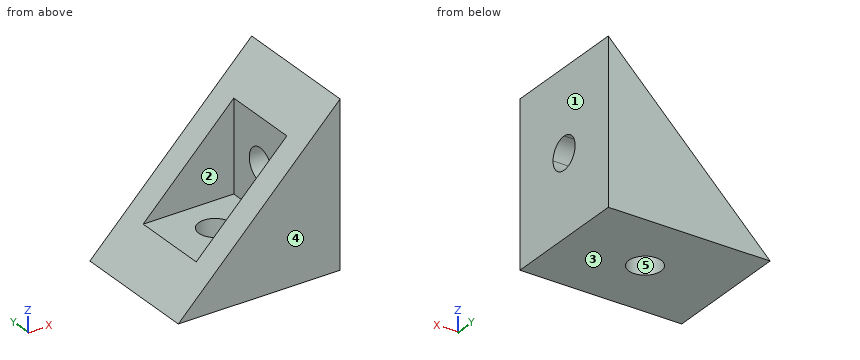
```python
from build123d import *

# Parameters (mm, degrees)
F1_DEPTH = 20
F2_DEPTH = 4
F4_DEPTH = 4
F6_DEPTH = 25.4
F7_R     = 2.5
F8_DEPTH = 25.4


with BuildPart() as f1:
    # F0 (on Front) → F1 (new body)
    with BuildSketch(Plane.XZ):
        Polygon((-7, -7), (-12.5, -12.5), (7, -12.5), (12.5, -12.5), (12.5, -7), (12.5, 12.5), (7, 7), (7, -7), align=None)
    extrude(amount=F1_DEPTH)

    # F0 (on Front) → F2 (join)
    with BuildSketch(Plane.XZ):
        Polygon((-7, -7), (-12.5, -12.5), (7, -12.5), (12.5, -12.5), (12.5, -7), (12.5, 12.5), (7, 7), (7, -7), align=None)
        Polygon((7, 7), (-7, -7), (7, -7), align=None)
    extrude(amount=F2_DEPTH)

    # F3 (on face) → F4 (join)
    with BuildSketch(Plane.XZ.offset(20)):
        Polygon((12.5, 12.5), (-12.5, -12.5), (12.5, -12.5), align=None)
    extrude(amount=-F4_DEPTH)

    # F5 (on face) → F6 (cut)
    with BuildSketch(Plane(origin=(7, 0, 0), x_dir=(0, -1, 0), z_dir=(-1, 0, 0))):
        with BuildLine():
            Line((10, 2.5), (10, -2.5))
            ThreePointArc((10, -2.5), (11.767767, -1.767767), (12.5, 0))
            ThreePointArc((12.5, 0), (11.767767, 1.767767), (10, 2.5))
        make_face()
        with BuildLine():
            ThreePointArc((10, 2.5), (7.5, 0), (10, -2.5))
            Line((10, -2.5), (10, 2.5))
        make_face()
    extrude(amount=-F6_DEPTH, mode=Mode.SUBTRACT)

    # F7 (on face) → F8 (cut)
    with BuildSketch(Plane.XY.offset(-7)):
        with Locations((0, -10)):
            Circle(F7_R)
    extrude(amount=-F8_DEPTH, mode=Mode.SUBTRACT)


solid = f1.part
```
The model under review builds one solid part; all positions refer to its coordinate system, in mm. Face numbers are marked on the shaded views. A direction names the side the tool comes from. Round coordinates to 2 decimals unless told otherwise and drop trailing zeros. Loops run counter-clockwise (first coordinate to the right, second up) from the corner with the lowest first, then second, coordinate; pieces in that order, holes last. Notation, with made-up numbers: M 70,-38.75 L 120,-38.75 A25 ccw 120,-24.75 Z; hole C 19.5,-11 d1. An arc over 180 degrees is marked long. Write item = value, one per line.
Item 1: Machinability: for the marked faces 1 and 2, which of the approach directions +Z, -Z, +X, -X, +Y, -Y give a long, thin tool a straight path to every point of the face, cutting with its end or side? Answer none if there is none.
Return value:
face_1 = +Z, -Z, +X, +Y, -Y
face_2 = +Z, -X
Item 2: Take a section at B-B on y = -9.5. Write out the cut boundary in (x, z), then the cut area to 3 significant figures.
Return value:
outline = M -12.5,-12.5 L -2.45,-12.5 L -2.45,-7 L -7,-7 Z; M 2.45,-12.5 L 12.5,-12.5 L 12.5,-2.45 L 7,-2.45 L 7,-7 L 2.45,-7 Z; M 7,2.45 L 12.5,2.45 L 12.5,12.5 L 7,7 Z
area = 161 mm2
Item 3: For line 1 (Y direction, x = 2.5, z = -2); line 2 (Y direction, x = 0, z = -11.15); line 3 (X direction, y = -7.25, z = -2), list the stretches that pass through material, from the lowest coordinate up. Write a range as [from, to].
Return value:
line_1 = [-20, -16], [-4, 0]
line_2 = [-20, -12.5], [-7.5, 0]
line_3 = [7, 12.5]
Item 4: Take a section at D-D on x = 5. Write out the cut boundary in (y, z), then the cut area to 3 significant figures.
Return value:
outline = M -20,-12.5 L 0,-12.5 L 0,5 L -4,5 L -4,-7 L -16,-7 L -16,5 L -20,5 Z
area = 206 mm2
Item 5: The part is to be moulded in two halves that separate along Y. For the marked faces 3, 4 and 5, say which applies: released by +Y, released by -Y, zero draft, split by the parting line, or undercut.
Return value:
face_3 = zero draft
face_4 = released by -Y
face_5 = undercut
Item 6: Take a section at A-A on x = 0. Write out the cut boundary in (y, z), then the cut area to 4 significant figures.
Return value:
outline = M -20,-12.5 L -12.5,-12.5 L -12.5,-7 L -16,-7 L -16,0 L -20,0 Z; M -7.5,-12.5 L 0,-12.5 L 0,0 L -4,0 L -4,-7 L -7.5,-7 Z
area = 138.5 mm2
Item 7: Insertion check: P1, Ø12, axis at x = -3, z = 3.5, coming from the -Y side; P2, Ø10, axis at x = -9, y = -12, coming from the +Z side; P3, Ø6, axis at y = -8, z = 3, coming from the -X side; P4, Ø8, axis at x = -5, z = 5.5, coming from the +Y side. Each pin has a flat end and moves straight along its axis. Give the tip position at first contact, or say it passes through.
Return value:
P1 = -20
P2 = -6
P3 = 7
P4 = through
Item 8: Take a section at C-C on z = 4.5. Write out the cut boundary in (x, y).
Return value:
outline = M 4.5,-20 L 12.5,-20 L 12.5,0 L 4.5,0 L 4.5,-4 L 7,-4 L 7,-16 L 4.5,-16 Z
